Autodesk Inventor part; units mm, degrees
ref_plane "YZ Plane" through (0, 0, 0) normal (1, 0, 0) x (0, 1, 0)
ref_plane "XZ Plane" through (0, 0, 0) normal (0, 1, 0) x (-1, 0, 0)
ref_plane "XY Plane" through (0, 0, 0) normal (0, 0, 1) x (1, 0, 0)
sketch "Sketch1" plane through (0, 0, 0) normal (0, 1, 0) x (-1, 0, 0)
  circle A0 centre (0, 0) radius 1.5
  line L0 (0, 3.1754) -> (2.75, 1.5877)
  line L1 (2.75, 1.5877) -> (2.75, -1.5877)
  line L2 (2.75, -1.5877) -> (0, -3.1754)
  line L3 (0, -3.1754) -> (-2.75, -1.5877)
  line L4 (-2.75, -1.5877) -> (-2.75, 1.5877)
  line L5 (-2.75, 1.5877) -> (0, 3.1754)
  dimension "d0" = 3
  dimension "d4" = 5.5
extrude "Extrusion1" add sketch "Sketch1" along normal blind 5
thread "Thread2"
sketch "Sketch3" plane through (0, 0, 0) normal (0, -1, 0) x (1, 0, 0)
  circle A0 centre (0, 0) radius 1.5066
extrude "Extrusion3" add sketch "Sketch3" along normal blind 6
thread "Thread3"
chamfer "Chamfer1" distance 0.3 angle 45 1 edges at (-1.5066, -6, 0)
properties part number "Spacer" material "Nylon 6"
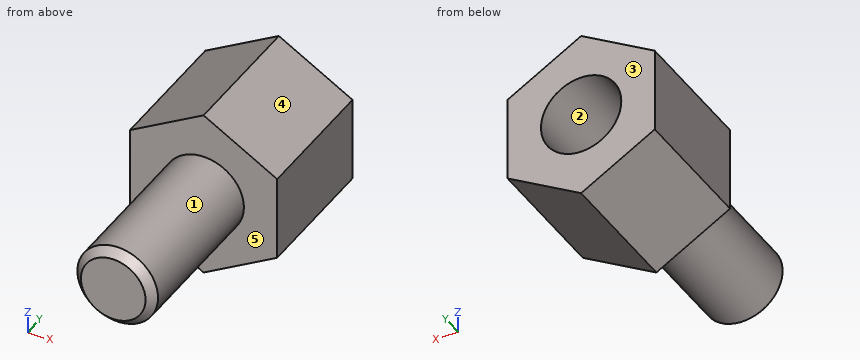
The model under review builds one solid part; all positions refer to its coordinate system, in mm. Face numbers are marked on the shaded views. A direction names the side the tool comes from. Give positions to 0.01 mm unless a question says otherwise; leave off trailing zeros. Write each loop counter-clockwise with the first axis right and the second up, starting at its lowest first coordinate (ties: lowest second). Pieces come first, ordered by that corner, then holes.
(1) To check wall thickness, follow L1, parallel to Y at x = 1.35, z = -2; L2, parallel to X at y = 0.75, z = -1; L3, parallel to Y at x = 0.35, z = -0.75. State the ranges of each line that lie inside material, in increasing order.
(2) Tool access review of the marked faces 4 and 5: name each direction out of +Z, -Z, +X, -X, +Y, -Y from which nothing blocks a thin tool from reaching the whole face with its end or side.
(3) For P1, Ø2, axis at x = 2, y = -3, coming from the +Z side, flat-tipped, find the tip position at first contact; note if it passes through.
(4) The part is to be moulded in two halves that separate along Z. For the marked faces 1, 2 and 3, say which applies: released by +Z, released by -Z, zero draft, split by the parting line, or undercut.
(5) Consider section A-A, the plane z = 0. Give the boundary of the cut face in (x, y).
(6) Consider section B-B, the plane y = -0.5. Give the boundary of the cut face in (x, z), and give its area (3 significant figures).
(7) Consider section C-C, the plane z = -2.5. Give the boundary of the cut face in (x, y).
Returned:
1. L1: y = 0 to 5
1. L2: x = -2.75 to -1.12, 1.12 to 2.75
1. L3: y = -6 to 0
2. face 4: +Z, +X, +Y, -Y
2. face 5: -Y
3. P1: stops at z = 1.13
4. face 1: split by the parting line
4. face 2: undercut
4. face 3: zero draft
5. outline: (-2.75, 0) - (-1.51, 0) - (-1.51, -5.7) - (-1.21, -6) - (1.21, -6) - (1.51, -5.7) - (1.51, 0) - (2.75, 0) - (2.75, 5) - (1.5, 5) - (1.5, 0) - (-1.5, 0) - (-1.5, 5) - (-2.75, 5) - close
6. outline: circle Ø3.01 at (0, 0)
6. area: 7.13 mm2
7. outline: (-1.17, 0) - (1.17, 0) - (1.17, 5) - (-1.17, 5) - close
